Work out the finished part from the listing and answer in its coordinate system (mm). A direction names the side the tool comes from. Give positions to 0.01 mm unless a question says otherwise; leave off trailing zeros. Loops run counter-clockwise (first coordinate to the right, second up) from the corner with the lowest first, then second, coordinate; pieces in that order, holes last. Notation, with made-up numbers: (23.25, -29.75) - (57.25, -29.75) arc R34 cw to (57.25, 6.25) - close; hole circle Ø5 at (26, -23). An arc over 180 degrees is marked (long way). One line per question, with ' | ' between items.
from build123d import *

# Parameters (mm, degrees)
BASE_FLANGE1_DEPTH = 63.5
SKETCH6_R          = 3.429
CUT_EXTRUDE1_DEPTH = 6.35
SKETCH7_R          = 20.32
CUT_EXTRUDE2_DEPTH = 6.35
SKETCH8_R          = 3.81
SKETCH8_R_2        = 3.831524444
CUT_EXTRUDE3_DEPTH = 6.35


# Read off the part's stored shape, not the designer's step: Base-Flange1
with BuildPart() as part:
    # Base-Flange1 outline → Base-Flange1 (new body)
    with BuildSketch(Plane.XY):
        with BuildLine():
            Line((48.14316, 19.56816), (48.14316, -127))
            Line((48.14316, -127), (50.8, -127))
            Line((50.8, -127), (50.8, 19.56816))
            ThreePointArc((50.8, 19.56816), (49.091893611, 23.691893611), (44.96816, 25.4))
            Line((44.96816, 25.4), (5.83184, 25.4))
            ThreePointArc((5.83184, 25.4), (1.708106389, 23.691893611), (0, 19.56816))
            Line((0, 19.56816), (0, 0))
            Line((0, 0), (2.65684, 0))
            Line((2.65684, 0), (2.65684, 19.56816))
            ThreePointArc((2.65684, 19.56816), (3.58677597, 21.81322403), (5.83184, 22.74316))
            Line((5.83184, 22.74316), (44.96816, 22.74316))
            ThreePointArc((44.96816, 22.74316), (47.21322403, 21.81322403), (48.14316, 19.56816))
        make_face()
    extrude(amount=BASE_FLANGE1_DEPTH)

    # Sketch6 → Cut-Extrude1 (cut)
    with BuildSketch(Plane.ZY):
        with Locations((6.35, 6.35)):
            Circle(SKETCH6_R)
        with Locations((57.15, 6.35)):
            Circle(SKETCH6_R)
    extrude(amount=-CUT_EXTRUDE1_DEPTH, mode=Mode.SUBTRACT)

    # Sketch7 → Cut-Extrude2 (cut)
    with BuildSketch(Plane(origin=(50.8, 0, 0), x_dir=(0, 0, -1), z_dir=(1, 0, 0))):
        with Locations(Location((-31.75, -93.46184, 0), (0, 0, 90))):
            Circle(SKETCH7_R)
    extrude(amount=-CUT_EXTRUDE2_DEPTH, mode=Mode.SUBTRACT)

    # Sketch8 → Cut-Extrude3 (cut)
    with BuildSketch(Plane(origin=(0, 25.4, 0), x_dir=(1, 0, 0), z_dir=(0, 1, 0))):
        with Locations(Location((9.9568, -12.699999998, 0), (0, 0, 270))):
            Circle(SKETCH8_R)
        with Locations(Location((9.9568, -50.799999998, 0), (0, 0, 270))):
            Circle(SKETCH8_R_2)
    extrude(amount=-CUT_EXTRUDE3_DEPTH, mode=Mode.SUBTRACT)


solid = part.part
1. Consider L1, parallel to Z at x = 1, y = 6; L2, parallel to X at y = 2, z = 39; L3, parallel to X at y = -74, z = 15. Determine where each line is inside the solid, lowest interval first.
Evaluation:
L1: 0 to 2.94, 9.76 to 53.74, 60.56 to 63.5 | L2: 0 to 2.66, 48.14 to 50.8 | L3: 48.14 to 50.8
2. Find section C-C on z = 14. Write down the section's boundary in (x, y) (3 decimals), then the cut area to 3 significant figures.
Evaluation:
outline: (0, 0) - (2.657, 0) - (2.657, 19.568) arc R3.175 cw to (5.832, 22.743) - (6.375, 22.743) - (6.375, 25.4) - (5.832, 25.4) arc R5.832 ccw to (0, 19.568) - close; (13.538, 22.743) - (44.968, 22.743) arc R3.175 cw to (48.143, 19.568) - (48.143, -83.57) - (50.8, -83.57) - (50.8, 19.568) arc R5.832 ccw to (44.968, 25.4) - (13.538, 25.4) - close; (48.143, -127) - (50.8, -127) - (50.8, -103.353) - (48.143, -103.353) - close | area: 511 mm2
3. Flat-ended cylindrical pins translate along their axes: pin 1 (19.5 mm diameter, centred on x = 21.5, z = 24.5, fed in from -Y); pin 2 (2 mm diameter, centred on y = -2.5, z = 43.5, fed in from -X); pin 3 (0.8 mm diameter, centred on x = 1, z = 35, fed in from -Y); pin 4 (8 mm diameter, centred on y = 6.35, z = 6.35, fed in from -X). Find the tip coordinate at first contact, or state that the pin passes through.
Evaluation:
pin 1: y = 22.74 | pin 2: x = 48.14 | pin 3: y = 0 | pin 4: x = 0
4. Find section B-B on z = 31.75. Write down the section's boundary in (x, y) (3 decimals), then the cut area to 3 significant figures.
Evaluation:
outline: (0, 0) - (2.657, 0) - (2.657, 19.568) arc R3.175 cw to (5.832, 22.743) - (44.968, 22.743) arc R3.175 cw to (48.143, 19.568) - (48.143, -73.142) - (50.8, -73.142) - (50.8, 19.568) arc R5.832 ccw to (44.968, 25.4) - (5.832, 25.4) arc R5.832 ccw to (0, 19.568) - close; (48.143, -127) - (50.8, -127) - (50.8, -113.782) - (48.143, -113.782) - close | area: 475 mm2
5. Which of the six approach directions +Z, -Z, +X, -X, +Y, -Y give full straight-line access (tool end or side, diameter ignored) to faces 5 (the cylindrical face through (1.31, 8.667, 54.623)), 6 (the flat face through (50.8, -55, 31)), 7 (the flat face through (48.143, -53, 31)), 8 (the flat face through (1, 0, 31))?
Evaluation:
face 5: -X | face 6: +Z, -Z, +X, +Y, -Y | face 7: +Z, -Z, -Y | face 8: +Z, -Z, -X, -Y
6. Find section D-D on x = 31. Write down the section's boundary in (y, z).
Evaluation:
outline: (22.74, 0) - (25.4, 0) - (25.4, 63.5) - (22.74, 63.5) - close
7. Determine the mould class of faces 1 (the cylindrical face through (1.31, 7.38, 9.62)), 2 (the cylindrical face through (49.137, 23.646, 31.306)), 3 (the cylindrical face through (49.5, -96.1, 51.9)), 4 (the cylindrical face through (10.125, 24.09, 46.972)) for opening direction Y: +Y half, -Y half, draft (parallel to the pull), parting line (faces both ways), or undercut.
Evaluation:
face 1: undercut | face 2: +Y half | face 3: undercut | face 4: draft
8. Find section A-A on y = 6.35. Write down the section's boundary in (x, z), then the cut area to 3 significant figures.
Evaluation:
outline: (0, 0) - (2.66, 0) - (2.66, 2.92) - (0, 2.92) - close; (0, 9.78) - (2.66, 9.78) - (2.66, 53.72) - (0, 53.72) - close; (0, 60.58) - (2.66, 60.58) - (2.66, 63.5) - (0, 63.5) - close; (48.14, 0) - (50.8, 0) - (50.8, 63.5) - (48.14, 63.5) - close | area: 301 mm2
